Autodesk Inventor part; units mm, degrees
ref_plane "YZ Plane" through (0, 0, 0) normal (1, 0, 0) x (0, 1, 0)
ref_plane "XZ Plane" through (0, 0, 0) normal (0, 1, 0) x (-1, 0, 0)
ref_plane "XY Plane" through (0, 0, 0) normal (0, 0, 1) x (1, 0, 0)
sketch "スケッチ1" plane through (0, 0, 0) normal (1, 0, 0) x (0, 1, 0)
  line L0 (-5, -5) -> (5, -5)
  line L1 (5, -5) -> (5, 5)
  line L2 (5, 5) -> (-5, 5)
  line L3 (-5, 5) -> (-5, -5)
  line L4 (-5, -5) -> (5, 5) construction
  line L5 (5, -5) -> (-5, 5) construction
  line L6 (4, 4) -> (4, -4)
  line L7 (4, -4) -> (-4, -4)
  line L8 (-4, -4) -> (-4, 4)
  line L9 (-4, 4) -> (4, 4)
  point P0 (0, 0)
  dimension "d0" = 1
  dimension "d1" = 10
  dimension "d2" = 10
extrude "押し出し1" add sketch "スケッチ1" along normal blind 30
sketch "スケッチ2" plane through (0, -5, 5) normal (0, 0, 1) x (1, 0, 0)
  line L0 (0, 5) -> (30, 5) construction
  line L1 (30, 9) -> (30, 1)
  circle A0 centre (7.5, 5) radius 1.5
  line L2 (0, 10) -> (0, 0)
  dimension "d5" = 3
  dimension "d6" = 7.5
extrude "押し出し2" cut sketch "スケッチ2" against normal through all
sketch "スケッチ3" plane through (0, 5, 5) normal (0, 1, 0) x (1, 0, 0)
  line L0 (0, 5) -> (30, 5) construction
  line L1 (30, 0) -> (30, 10)
  circle A0 centre (22.5, 5) radius 1.5
  dimension "d9" = 3
  dimension "d10" = 7.5
extrude "押し出し3" cut sketch "スケッチ3" against normal through all
sketch "スケッチ4" plane through (0, 5, 5) normal (0, 1, 0) x (1, 0, 0)
  line L0 (30, 10) -> (30, 0)
  line L1 (0, 10) -> (0, 0)
  circle A0 centre (22.5, 5) radius 1.5
  point P0 (0, 5)
  dimension "d13" = 30
  dimension "d14" = 22.5
sketch "スケッチ5" plane through (0, -5, 5) normal (0, 0, 1) x (1, 0, 0)
  line L0 (30, 10) -> (30, 0)
  line L1 (0, 10) -> (0, 0)
  circle A0 centre (7.5, 5) radius 1.5
  point P0 (0, 5)
  dimension "d16" = 7.5
properties part number "omu_k_jo_5" material "アルミニウム 6061-AHC"
Source: CAD feature listing. Evaluate the final solid. Frame: model axes, mm. A direction names the side the tool comes from. Round coordinates to 2 decimals unless told otherwise and drop trailing zeros. Write each loop counter-clockwise with the first axis right and the second up, starting at its lowest first coordinate (ties: lowest second). Pieces come first, ordered by that corner, then holes. Notation, with made-up numbers: (-12.75, 72.5) - (34.25, 72.5) arc R20 cw to (34.25, 85.5) - close; hole circle Ø1 at (59, -33). An arc over 180 degrees is marked (long way). Use CSV: the item, a comma, the result in double quotes. Start each with the question number.
(1) Mould query, pull axis Y, two halves, no side actions, for faces 1 (the face through (15, -5, 0)), 2 (the face through (6, 0.07, -4.49)), 3 (the face through (21, -4.49, -0.07)). Classes: pulls with the +Y half, pulls with the -Y half, needs draft (parallel to the pull), parting line crosses it, or undercut.
(2) Material intervals for probe 1 along Z at (x, y) = (22.5, -4.2); probe 2 along Z at (x, y) = (27.5, 3); probe 3 along X at (y, z) = (4.6, 0), sorted ascending. Write a range as [from, to].
(3) Cut plane D-D, the plane z = -2. Return loops of the section in (x, y), and give its area (3 significant figures).
(4) Cut plane A-A, the plane x = 7.5. Return loops of the section in (y, z).
(5) Cut plane C-C, the plane z = 0. Return loops of the section in (x, y), and give its area (3 significant figures).
(6) Set-up query: faces 4 (the face through (15, 0, -4)), 5 (the face through (15, 0, 5)). Return all of +Z, -Z, +X, -X, +Y, -Y with unobstructed straight access to the full face (end or side cutting, diameter ignored); none if empty.
(7) Cut plane B-B, the plane y = 0. Return loops of the section in (x, z), and give its area (3 significant figures).
(8) First-contact query: pin 1 Ø4 at (x, z) = (22.5, 0) entering from +Y; pin 2 Ø1.5 at (y, z) = (1.5, -2.5) entering from +X. Flat tips, straight axial feed; report the tip coordinate or a pass-through.
Geometry says:
1,face 1,"pulls with the -Y half"
1,face 2,"undercut"
1,face 3,"needs draft"
2,probe 1,"[-5, -1.5], [1.5, 5]"
2,probe 2,"[-5, -4], [4, 5]"
2,probe 3,"[0, 21], [24, 30]"
3,outline,"(0, -5) - (30, -5) - (30, -4) - (0, -4) - close; (0, 4) - (30, 4) - (30, 5) - (0, 5) - close"
3,area,"60.0 mm²"
4,outline,"(-5, -5) - (-1.5, -5) - (-1.5, -4) - (-4, -4) - (-4, 4) - (-1.5, 4) - (-1.5, 5) - (-5, 5) - close; (1.5, -5) - (5, -5) - (5, 5) - (1.5, 5) - (1.5, 4) - (4, 4) - (4, -4) - (1.5, -4) - close"
5,outline,"(0, -5) - (21, -5) - (21, -4) - (0, -4) - close; (0, 4) - (21, 4) - (21, 5) - (0, 5) - close; (24, -5) - (30, -5) - (30, -4) - (24, -4) - close; (24, 4) - (30, 4) - (30, 5) - (24, 5) - close"
5,area,"54.0 mm²"
6,face 4,"+X, -X"
6,face 5,"+Z, +X, -X, +Y, -Y"
7,outline,"(0, -5) - (6, -5) - (6, -4) - (0, -4) - close; (0, 4) - (6, 4) - (6, 5) - (0, 5) - close; (9, -5) - (30, -5) - (30, -4) - (9, -4) - close; (9, 4) - (30, 4) - (30, 5) - (9, 5) - close"
7,area,"54.0 mm²"
8,pin 1,"y = 5"
8,pin 2,"through"
